Build history of the part. All positions in model axes, mm. A direction names the side the tool comes from. Round coordinates to 2 decimals unless told otherwise and drop trailing zeros. Loops run counter-clockwise (first coordinate to the right, second up) from the corner with the lowest first, then second, coordinate; pieces in that order, holes last. Notation, with made-up numbers: (43, 71.5) - (66, 71.5) arc R31 ccw to (66, 99.5) - close; hole circle Ø10 at (-28.75, 49.5). An arc over 180 degrees is marked (long way). Use a Markdown table: item, result.
from build123d import *

# Parameters (mm, degrees)
SKETCH1_W            = 195
SKETCH1_H            = 205
BOSS_EXTRUDE1_DEPTH  = 5
CUT_EXTRUDE2_DEPTH   = 228.060014093
SKETCH6_W            = 10
SKETCH6_H            = 48
SKETCH6_W_2          = 48
SKETCH6_H_2          = 10
BOSS_EXTRUDE3_DEPTH  = 4
SKETCH11_R           = 1.75
RETAINER_HOLES_DEPTH = 228.060014093
SKETCH14_R           = 3.25
HANDLE_MOUNT_DEPTH   = 228.060014093
SKETCH12_W           = 10
SKETCH12_H           = 130
RIBS_DEPTH           = 5


with BuildPart() as part:
    # Sketch1 → Boss-Extrude1 (new body)
    with BuildSketch(Plane.XY):
        with Locations((0, -102.5)):
            Rectangle(SKETCH1_W, SKETCH1_H)
    extrude(amount=BOSS_EXTRUDE1_DEPTH)

    # Sketch5 → Cut-Extrude2 (cut, through all)
    with BuildSketch(Plane.XY.offset(5)):
        Polygon((-25, -83.25), (37, -83.25), (37, -188.25), (-63, -188.25), (-63, -163.25), (-25, -163.25), align=None)
        Polygon((88.25, -113), (63.25, -113), (63.25, -75), (-16.75, -75), (-16.75, -13), (88.25, -13), align=None)
    extrude(amount=-CUT_EXTRUDE2_DEPTH, mode=Mode.SUBTRACT)

    # Sketch6 → Boss-Extrude3 (add)
    with BuildSketch(Plane(origin=(0, 0, 0), x_dir=(-1, 0, 0), z_dir=(0, 0, -1))):
        with Locations((20, -139.25)):
            Rectangle(SKETCH6_W, SKETCH6_H)
        Polygon((23, -188.25), (23, -182.25), (-27, -182.25), (-27, -115.25), (-37, -115.25), (-37, -188.25), align=None)
        Polygon((-88.25, -73), (-82.25, -73), (-82.25, -23), (-15.25, -23), (-15.25, -13), (-88.25, -13), align=None)
        with Locations((-39.25, -70)):
            Rectangle(SKETCH6_W_2, SKETCH6_H_2)
    extrude(amount=-BOSS_EXTRUDE3_DEPTH)

    # Sketch11 → Retainer Holes (cut, through all)
    with BuildSketch(Plane.XY.offset(5)):
        with Locations((42, -153.25)):
            Circle(SKETCH11_R)
        with Locations((42, -178.25)):
            Circle(SKETCH11_R)
        with Locations((-30, -150.75)):
            Circle(SKETCH11_R)
        with Locations((50.75, -80)):
            Circle(SKETCH11_R)
        with Locations((53.25, -8)):
            Circle(SKETCH11_R)
        with Locations((78.25, -8)):
            Circle(SKETCH11_R)
    extrude(amount=-RETAINER_HOLES_DEPTH, mode=Mode.SUBTRACT)

    # Sketch14 → Handle Mount (cut, through all)
    with BuildSketch(Plane.XY.offset(5)):
        with Locations((-50, -197)):
            Circle(SKETCH14_R)
        with Locations((50, -197)):
            Circle(SKETCH14_R)
        with Locations((0, -197)):
            Circle(SKETCH14_R)
    extrude(amount=-HANDLE_MOUNT_DEPTH, mode=Mode.SUBTRACT)

    # Sketch12 → Ribs (add)
    with BuildSketch(Plane.XY.offset(5)):
        with Locations((-40, -75)):
            Rectangle(SKETCH12_W, SKETCH12_H)
    extrude(amount=RIBS_DEPTH)


solid = part.part
Q1. Cut at C-C, the plane y = -95. List the corners of the cut face in (x, z).
Results found:
| item | result |
|---|---|
| outline | (-97.5, 0) - (-25, 0) - (-25, 5) - (-35, 5) - (-35, 10) - (-45, 10) - (-45, 5) - (-97.5, 5) - close; (37, 0) - (63.25, 0) - (63.25, 5) - (37, 5) - close; (88.25, 0) - (97.5, 0) - (97.5, 5) - (88.25, 5) - close |
Q2. Probe line 1 (Y direction, x = 0, z = 2.65); line 2 (Y direction, x = -6, z = 1); line 3 (X direction, y = -94, z = 3.5). List the from-to ranges inside material, lowest first.
Results found:
| item | result |
|---|---|
| line 1 | y = -205 to -200.25, -193.75 to -182.25, -83.25 to -75, -13 to 0 |
| line 2 | y = -205 to -182.25, -83.25 to -75, -13 to 0 |
| line 3 | x = -97.5 to -25, 37 to 63.25, 88.25 to 97.5 |
Q3. Cut at D-D, the plane z = 7.5. List the corners of the cut face in (x, y), plus the area to 3 significant figures.
Results found:
| item | result |
|---|---|
| outline | (-45, -140) - (-35, -140) - (-35, -10) - (-45, -10) - close |
| area | 1,300 mm2 |
Q4. Which spindle directions (+Z, -Z, +X, -X, +Y, -Y) get a long thin tool onto all of the face, cutting with end or side? Do faces 5 (the face through (-20, -124, 0)), 6 (the face through (-39, -163.25, 2)), 7 (the face through (-1, 0, 2)), 8 (the face through (-45, -76, 7)), 9 (the face through (-35, -188.25, 3)). Say none if no direction does.
Results found:
| item | result |
|---|---|
| face 5 | -Z, +X, -X, +Y, -Y |
| face 6 | +Z, -Z |
| face 7 | +Z, -Z, +X, -X, +Y |
| face 8 | +Z, -X, +Y, -Y |
| face 9 | +Z |
Q5. Drop flat-ended pins along their axis: pin 1 (8 mm diameter, centred on x = -61, y = -98.5, fed in from -Z); pin 2 (8.5 mm diameter, centred on x = -50, y = -197, fed in from +Z); pin 3 (2 mm diameter, centred on y = -23.5, z = 8, fed in from +X); pin 4 (18 mm diameter, centred on x = 52, y = -31.5, fed in from +Z). Give the stop position or say it passes through.
Results found:
| item | result |
|---|---|
| pin 1 | stops at z = 0 |
| pin 2 | stops at z = 5 |
| pin 3 | stops at x = -35 |
| pin 4 | stops at z = 4 |
Q6. Cut at B-B, the plane y = -125. List the corners of the cut face in (x, z), plus the area to 3 significant figures.
Results found:
| item | result |
|---|---|
| outline | (-97.5, 0) - (-15, 0) - (-15, 4) - (-25, 4) - (-25, 5) - (-35, 5) - (-35, 10) - (-45, 10) - (-45, 5) - (-97.5, 5) - close; (27, 0) - (97.5, 0) - (97.5, 5) - (37, 5) - (37, 4) - (27, 4) - close |
| area | 795 mm2 |
Q7. Pull direction Y, two halves, no side cores. Call faces 1 (the face through (63, -21, 4)), 2 (the face through (-40, -74, 10)), 3 (the face through (-40, -140, 7)), 4 (the face through (12, -13, 3)): pulls with the +Y half, pulls with the -Y half, needs draft (parallel to the pull), parting line crosses it, or undercut.
Results found:
| item | result |
|---|---|
| face 1 | undercut |
| face 2 | needs draft |
| face 3 | pulls with the -Y half |
| face 4 | undercut |
Q8. Cut at A-A, the plane x = 0. List the corners of the cut face in (y, z).
Results found:
| item | result |
|---|---|
| outline | (-205, 0) - (-200.25, 0) - (-200.25, 5) - (-205, 5) - close; (-193.75, 0) - (-182.25, 0) - (-182.25, 4) - (-188.25, 4) - (-188.25, 5) - (-193.75, 5) - close; (-83.25, 0) - (-75, 0) - (-75, 5) - (-83.25, 5) - close; (-13, 0) - (0, 0) - (0, 5) - (-13, 5) - close |
